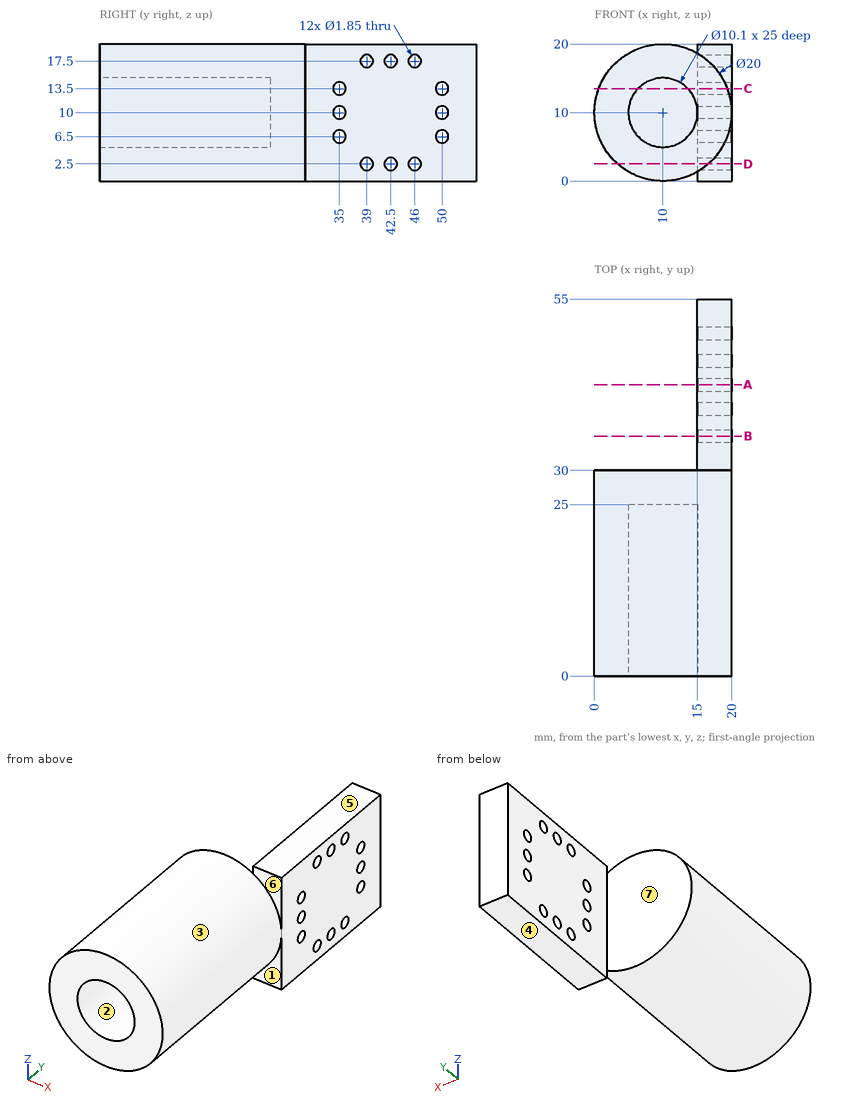
Print and shaded views of the part. All mm, measured from the part's lowest x, y and z. A direction names the side the tool comes from. Give positions to 0.01 mm unless a question says otherwise; leave off trailing zeros. Order: outer loops, then holes, each group sorted by start corner. A loop starts at its lowest first (then second) coordinate and runs counter-clockwise, first axis right, second up. Notation, with made-up numbers: M -6.5,28 L 9.5,28 A25 ccw 9.5,56 Z; hole C 22.5,69 d3. An arc over 180 degrees is marked long. Use one line per item in the form item = value.
Q1. Pull direction Z, two halves, no side cores. Call the marked faces 1, 2, 3 and 4: released by +Z, released by -Z, zero draft, split by the parting line, or undercut.
Conclusion:
face_1 = zero draft
face_2 = undercut
face_3 = split by the parting line
face_4 = released by -Z
Q2. Wall check: probe 1 along Y at (x, z) = (16.9, 6.5) (3 decimals); probe 2 along Z at (x, y) = (18.15, 35) (3 decimals); probe 3 along Y at (x, z) = (17.9, 2.5) (3 decimals). Give the ranges that are in metal, low to high.
Conclusion:
probe_1 = 0 to 34.075, 35.925 to 49.075, 50.925 to 55
probe_2 = 0 to 5.575, 7.425 to 9.075, 10.925 to 12.575, 14.425 to 20
probe_3 = 30 to 38.075, 39.925 to 41.575, 43.425 to 45.075, 46.925 to 55
Q3. Slice it at A-A, the plane y = 42.5. Write the cut outline in (x, z) (3 decimals).
Conclusion:
outline = M 15,0 L 20,0 L 20,1.575 L 15,1.575 Z; M 15,3.425 L 20,3.425 L 20,16.575 L 15,16.575 Z; M 15,18.425 L 20,18.425 L 20,20 L 15,20 Z
Q4. Slice it at D-D, the plane z = 2.5. Write the cut outline in (x, y) (3 decimals), and give its area (3 significant figures).
Conclusion:
outline = M 3.386,0 L 16.614,0 L 16.614,30 L 20,30 L 20,38.075 L 15,38.075 L 15,30 L 3.386,30 Z; M 15,39.925 L 20,39.925 L 20,41.575 L 15,41.575 Z; M 15,43.425 L 20,43.425 L 20,45.075 L 15,45.075 Z; M 15,46.925 L 20,46.925 L 20,55 L 15,55 Z
area = 494 mm2
Q5. Which spindle directions (+Z, -Z, +X, -X, +Y, -Y) get a long thin tool onto all of the face, cutting with end or side? Do the marked faces 5, 6 and 7. Say none if no direction does.
Conclusion:
face_5 = +Z, +X, -X, +Y, -Y
face_6 = +Z, +X, -Y
face_7 = +Z, -Z, -X, +Y
Q6. Pin check, flat tips, straight feed: P1, Ø3, axis at x = 11, z = 5.5, coming from the +Y side; P2, Ø1.7, axis at y = 42.5, z = 17.5, coming from the +X side; P3, Ø1.5, axis at x = 18.5, z = 2.5, coming from the -Y side; P4, Ø4, axis at y = 7.5, z = 4, coming from the -X side. Stop position of each tip, or through.
Conclusion:
P1 = 30
P2 = through
P3 = 30
P4 = 0.83
Q7. Slice it at C-C, the plane z = 13.5. Write the cut outline in (x, y) (1 decimal), and give its area (3 significant figures).
Conclusion:
outline = M 0.6,0 L 6.4,0 L 6.4,25 L 13.6,25 L 13.6,0 L 19.4,0 L 19.4,30 L 20,30 L 20,34.1 L 15,34.1 L 15,30 L 0.6,30 Z; M 15,35.9 L 20,35.9 L 20,49.1 L 15,49.1 Z; M 15,50.9 L 20,50.9 L 20,55 L 15,55 Z
area = 487 mm2
Q8. Slice it at B-B, the plane y = 35. Write the cut outline in (x, z) (3 decimals), and give its area (4 significant figures).
Conclusion:
outline = M 15,0 L 20,0 L 20,5.575 L 15,5.575 Z; M 15,7.425 L 20,7.425 L 20,9.075 L 15,9.075 Z; M 15,10.925 L 20,10.925 L 20,12.575 L 15,12.575 Z; M 15,14.425 L 20,14.425 L 20,20 L 15,20 Z
area = 72.25 mm2
